For this review, take the finished solid that the model builds, in its own axes (mm). A direction names the side the tool comes from. Round coordinates to 2 decimals unless told otherwise and drop trailing zeros. Order: outer loops, then holes, each group sorted by start corner. A loop starts at its lowest first (then second) coordinate and runs counter-clockwise, first axis right, second up. Notation, with made-up numbers: (-22.5, -20.5) -> (31.5, -20.5) arc R13 cw to (31.5, 3.5) -> close; hole circle Ø11 at (16.25, 30.25). An arc over 180 degrees is marked (long way). Answer in a Markdown table with one row per item.
```python
from build123d import *

# Parameters (mm, degrees)
BOSS_EXTRUDE4_DEPTH = 60
CUT_EXTRUDE2_DEPTH  = 60
SKETCH8_R           = 2.5
CUT_EXTRUDE3_DEPTH  = 60
CUT_EXTRUDE4_START  = 25.5
CUT_EXTRUDE4_DEPTH  = 9
SKETCH10_W          = 43.881633461
SKETCH10_H          = 22.720590432
CUT_EXTRUDE5_DEPTH  = 20
SKETCH11_W          = 44.457178834
SKETCH11_H          = 22.765793249
CUT_EXTRUDE6_DEPTH  = 20
FILLET1_R           = 5
FILLET2_R           = 5
FILLET3_R           = 5
FILLET4_R           = 5
CUT_EXTRUDE7_DEPTH  = 49
CUT_EXTRUDE8_DEPTH  = 15
CUT_EXTRUDE9_DEPTH  = 45
CUT_EXTRUDE10_DEPTH = 18
SKETCH14_R          = 1.5
CUT_EXTRUDE11_DEPTH = 20
SKETCH15_R          = 1.5
CUT_EXTRUDE12_DEPTH = 20
SKETCH16_R          = 1.5
CUT_EXTRUDE13_DEPTH = 20
SKETCH17_R          = 1.5
CUT_EXTRUDE14_DEPTH = 20
SKETCH18_R          = 1.5
CUT_EXTRUDE15_DEPTH = 20
SKETCH19_R          = 1.5
CUT_EXTRUDE16_DEPTH = 15
SKETCH20_R          = 1.5
CUT_EXTRUDE17_DEPTH = 15


with BuildPart() as part:
    # Sketch5 → Boss-Extrude4 (new body)
    with BuildSketch(Plane.XY):
        with BuildLine():
            Line((-5.591433469, 0), (-33.737961989, 0))
            ThreePointArc((-33.737961989, 0), (-37.261513388, 1.45252406), (-38.737847513, 4.966165783))
            ThreePointArc((-38.737847513, 4.966165783), (-31.616240623, 53.699065918), (-10.244585549, 98.070962427))
            ThreePointArc((-10.244585549, 98.070962427), (-7.858330599, 99.704279242), (-4.994698694, 99.302347885))
            ThreePointArc((-4.994698694, 99.302347885), (-1.130402236, 95.400824643), (0.061459935, 90.040401592))
            ThreePointArc((0.061459935, 90.040401592), (-0.013962808, 89.477441364), (-0.168362399, 88.93083952))
            ThreePointArc((-0.168362399, 88.93083952), (-7.882068029, 47.204430035), (-1.77951237, 5.212129342))
            ThreePointArc((-1.77951237, 5.212129342), (-2.362771411, 1.638699232), (-5.591433469, 0))
        make_face()
        Polygon((-23.793249775, 26.029552985), (-22.148877555, 31.130017156), (-25.743822989, 35.104317357), (-30.983140641, 33.978153386), (-32.627512861, 28.877689216), (-29.032567427, 24.903389015), align=None, mode=Mode.SUBTRACT)
        Polygon((-19.704548153, 50.537737556), (-20.448711238, 55.006105989), (-24.690513357, 56.595826069), (-28.18815239, 53.717177716), (-27.443989306, 49.248809284), (-23.202187187, 47.659089203), align=None, mode=Mode.SUBTRACT)
        Polygon((-12.020901099, 69.614378519), (-12.60140651, 74.617120781), (-17.224161103, 76.615759479), (-21.266410285, 73.611655915), (-20.685904874, 68.608913653), (-16.063150281, 66.610274955), align=None, mode=Mode.SUBTRACT)
        Polygon((-4.994698694, 87.366252749), (-5.009667304, 90.521352685), (-7.749548306, 92.085939457), (-10.474460698, 90.495426291), (-10.459492087, 87.340326355), (-7.719611085, 85.775739583), align=None, mode=Mode.SUBTRACT)
        Polygon((-12.020901099, 37.637700147), (-12.875266359, 41.812019441), (-16.917515541, 43.159277068), (-20.105399463, 40.332215402), (-19.251034203, 36.157896108), (-15.208785021, 34.810638481), align=None, mode=Mode.SUBTRACT)
        Polygon((-12.020901099, 55.800966029), (-10.82059125, 58.827758896), (-12.841715841, 61.380654151), (-16.063150281, 60.906756539), (-17.263460129, 57.879963671), (-15.242335538, 55.327068416), align=None, mode=Mode.SUBTRACT)
    extrude(amount=BOSS_EXTRUDE4_DEPTH)

    # Sketch7 → Cut-Extrude2 (cut)
    with BuildSketch(Plane.XY.offset(60)):
        with BuildLine():
            Line((-12, 7.5121344), (-7, 7.5121344))
            ThreePointArc((-7, 7.5121344), (-4.4878656, 5), (-7, 2.4878656))
            Line((-7, 2.4878656), (-12, 2.4878656))
            ThreePointArc((-12, 2.4878656), (-14.5121344, 5), (-12, 7.5121344))
        make_face()
    extrude(amount=-CUT_EXTRUDE2_DEPTH, mode=Mode.SUBTRACT)

    # Sketch8 → Cut-Extrude3 (cut)
    with BuildSketch(Plane.XY.offset(60)):
        with Locations((-32.283791832, 6.170765259)):
            Circle(SKETCH8_R)
    extrude(amount=-CUT_EXTRUDE3_DEPTH, mode=Mode.SUBTRACT)

    # Sketch9 → Cut-Extrude4 (cut)
    with BuildSketch(Plane.XY.offset(CUT_EXTRUDE4_START)):
        with BuildLine():
            Line((0, 0), (-18.287002555, 0))
            ThreePointArc((-18.287002555, 0), (-19.970817175, 0.920755669), (-20.104249938, 2.835231673))
            Line((-20.104249938, 2.835231673), (-7.17958851, 30.955941067))
            Line((-7.17958851, 30.955941067), (0, 0))
        make_face()
    extrude(amount=CUT_EXTRUDE4_DEPTH, mode=Mode.SUBTRACT)

    # Sketch10 → Cut-Extrude5 (cut)
    with BuildSketch(Plane(origin=(0, 0, 0), x_dir=(-1, 0, 0), z_dir=(0, 0, -1))):
        with Locations((18.890622206, 8.639704784)):
            Rectangle(SKETCH10_W, SKETCH10_H)
    extrude(amount=-CUT_EXTRUDE5_DEPTH, mode=Mode.SUBTRACT)

    # Sketch11 → Cut-Extrude6 (cut)
    with BuildSketch(Plane.XY.offset(60)):
        with Locations((-18.356989611, 8.617103375)):
            Rectangle(SKETCH11_W, SKETCH11_H)
    extrude(amount=-CUT_EXTRUDE6_DEPTH, mode=Mode.SUBTRACT)

    # Fillet1
    fillet1_edges = [part.edges().sort_by_distance(p)[0] for p in [
        (-5.544200811, 20, 50),
    ]]
    fillet(fillet1_edges, radius=FILLET1_R)

    # Fillet2
    fillet2_edges = [part.edges().sort_by_distance(p)[0] for p in [
        (-5.544200811, 20, 10),
    ]]
    fillet(fillet2_edges, radius=FILLET2_R)

    # Fillet3
    fillet3_edges = [part.edges().sort_by_distance(p)[0] for p in [
        (-38.144186452, 20, 50),
    ]]
    fillet(fillet3_edges, radius=FILLET3_R)

    # Fillet4
    fillet4_edges = [part.edges().sort_by_distance(p)[0] for p in [
        (-38.144186452, 20, 10),
    ]]
    fillet(fillet4_edges, radius=FILLET4_R)

    # Sketch12 → Cut-Extrude7 (cut)
    with BuildSketch(Plane(origin=(0, 0, 0), x_dir=(0, 0, -1), z_dir=(1, 0, 0))):
        Polygon((-60, 20), (-60, 99.809969504), (-40, 99.809969504), align=None)
    extrude(amount=-CUT_EXTRUDE7_DEPTH, mode=Mode.SUBTRACT)

    # Sketch12<2> → Cut-Extrude8 (cut)
    with BuildSketch(Plane(origin=(0, 0, 0), x_dir=(0, 0, -1), z_dir=(1, 0, 0))):
        Polygon((-60, 20), (-60, 99.809969504), (-40, 99.809969504), align=None)
    extrude(amount=CUT_EXTRUDE8_DEPTH, mode=Mode.SUBTRACT)

    # Sketch13 → Cut-Extrude9 (cut)
    with BuildSketch(Plane(origin=(0, 0, 0), x_dir=(0, 0, -1), z_dir=(1, 0, 0))):
        Polygon((0, 20), (0, 99.809969504), (-20, 99.809969504), align=None)
    extrude(amount=-CUT_EXTRUDE9_DEPTH, mode=Mode.SUBTRACT)

    # Sketch13<2> → Cut-Extrude10 (cut)
    with BuildSketch(Plane(origin=(0, 0, 0), x_dir=(0, 0, -1), z_dir=(1, 0, 0))):
        Polygon((0, 20), (0, 99.809969504), (-20, 99.809969504), align=None)
    extrude(amount=CUT_EXTRUDE10_DEPTH, mode=Mode.SUBTRACT)

    # Sketch14 → Cut-Extrude11 (cut)
    with BuildSketch(Plane(origin=(0, 0, 0), x_dir=(0, 0, -1), z_dir=(1, 0, 0))):
        with Locations((-49.873134451, 35.727910902)):
            Circle(SKETCH14_R)
    extrude(amount=-CUT_EXTRUDE11_DEPTH, mode=Mode.SUBTRACT)

    # Sketch15 → Cut-Extrude12 (cut)
    with BuildSketch(Plane(origin=(0, 0, 0), x_dir=(0, 0, -1), z_dir=(1, 0, 0))):
        with Locations((-30.002133338, 35.727910902)):
            Circle(SKETCH15_R)
    extrude(amount=-CUT_EXTRUDE12_DEPTH, mode=Mode.SUBTRACT)

    # Sketch16 → Cut-Extrude13 (cut)
    with BuildSketch(Plane(origin=(0, 0, 0), x_dir=(0, 0, -1), z_dir=(1, 0, 0))):
        with Locations((-10.126865549, 35.727910902)):
            Circle(SKETCH16_R)
    extrude(amount=-CUT_EXTRUDE13_DEPTH, mode=Mode.SUBTRACT)

    # Sketch17 → Cut-Extrude14 (cut)
    with BuildSketch(Plane(origin=(0, 0, 0), x_dir=(0, 0, -1), z_dir=(1, 0, 0))):
        with Locations((-44.360038747, 57.727910902)):
            Circle(SKETCH17_R)
    extrude(amount=-CUT_EXTRUDE14_DEPTH, mode=Mode.SUBTRACT)

    # Sketch18 → Cut-Extrude15 (cut)
    with BuildSketch(Plane(origin=(0, 0, 0), x_dir=(0, 0, -1), z_dir=(1, 0, 0))):
        with Locations((-15.639961253, 57.727910902)):
            Circle(SKETCH18_R)
    extrude(amount=-CUT_EXTRUDE15_DEPTH, mode=Mode.SUBTRACT)

    # Sketch19 → Cut-Extrude16 (cut)
    with BuildSketch(Plane(origin=(0, 0, 0), x_dir=(0, 0, -1), z_dir=(1, 0, 0))):
        with Locations((-37.793709057, 83.93083952)):
            Circle(SKETCH19_R)
    extrude(amount=-CUT_EXTRUDE16_DEPTH, mode=Mode.SUBTRACT)

    # Sketch20 → Cut-Extrude17 (cut)
    with BuildSketch(Plane(origin=(0, 0, 0), x_dir=(0, 0, -1), z_dir=(1, 0, 0))):
        with Locations((-22.206290943, 83.93083952)):
            Circle(SKETCH20_R)
    extrude(amount=-CUT_EXTRUDE17_DEPTH, mode=Mode.SUBTRACT)


solid = part.part
```
Q1. Tool access review of faces 1 (the face through (-20.07, 52.74, 29.69)), 2 (the face through (-2.332, 1.681, 37.212)), 3 (the face through (-15, 84, 22)): name each direction out of +Z, -Z, +X, -X, +Y, -Y from which nothing blocks a thin tool from reaching the whole face with its end or side.
Answer key:
| item | result |
|---|---|
| face 1 | +Z, -Z |
| face 2 | +Z, -Z, +X |
| face 3 | +X |
Q2. To check wall thickness, follow probe 1 along Y at (x, z) = (-14, 23); probe 2 along Y at (x, z) = (-9, 23.5); probe 3 along X at (y, z) = (67, 38.5). State the ranges of each line that lie inside material, in increasing order.
Answer key:
| item | result |
|---|---|
| probe 1 | y = 0 to 3.48, 6.52 to 35.88, 42.19 to 55.51, 61.21 to 68.14, 75.22 to 82.66, 85.2 to 92.33 |
| probe 2 | y = 0 to 2.49, 7.51 to 83.17, 84.69 to 86.51, 91.36 to 99.24 |
| probe 3 | x = -26.91 to -16.96, -15.54 to -5.98 |
Q3. Take a section at A-A, the plane y = 23. Write out the cut boundary in (x, z), then the cut area to 3 significant figures.
Answer key:
| item | result |
|---|---|
| outline | (-37.86, 20) -> (-37.18, 20) -> (-37.18, 0.75) -> (-6.88, 0.75) -> (-6.88, 20) -> (-6.09, 20) -> (-6.09, 25.5) -> (-10.84, 25.5) -> (-10.84, 34.5) -> (-6.09, 34.5) -> (-6.09, 40) -> (-6.88, 40) -> (-6.88, 59.25) -> (-37.18, 59.25) -> (-37.18, 40) -> (-37.86, 40) -> close |
| area | 1,760 mm^2 |
Q4. Clearance check with flat-ended pins moving along their axes: pin 1 Ø20.5 at (x, y) = (-10, 9.5) entering from -Z; pin 2 Ø5.5 at (x, y) = (-13.5, 11) entering from +Z; pin 3 Ø1.8 at (y, z) = (35.73, 49.87) entering from -X. State where each tip first meets the part, or that it passes through.
Answer key:
| item | result |
|---|---|
| pin 1 | stops at z = 20 |
| pin 2 | stops at z = 40 |
| pin 3 | stops at x = -36.18 |
Q5. The part is to be moulded in two halves that separate along X. For faces 4 (the face through (-20, 36, 10)), 5 (the face through (-19.217, 75.135, 29.768)), say which applies: +X half, -X half, draft (parallel to the pull), parting line (faces both ways), or undercut.
Answer key:
| item | result |
|---|---|
| face 4 | +X half |
| face 5 | undercut |
